Could you check a few things on this model? Use its own coordinates, in mm. Face numbers are marked on the shaded views. Round coordinates to 2 decimals unless told otherwise and drop trailing zeros. Order: outer loops, then holes, each group sorted by start corner. A loop starts at its lowest first (then second) coordinate and runs counter-clockwise, first axis right, second up. Notation, with made-up numbers: M 22,37 L 41,37 A37 cw 41,74 Z; hole C 51,74 d5. An arc over 180 degrees is marked long. Write each question's results on one line, items separated by ' | '. Start each with the question number.
1. Please list where these lines run through material, in increasing order: L1, parallel to Y at x = 0, z = 1.95; L2, parallel to Y at x = -2.25, z = 0.4; L3, parallel to Z at x = -3.75, y = 2.
2. We'd pull the mould along X, two halves only. Please class the marked faces 1, 2 and 3: released by +X, released by -X, zero draft, split by the parting line, or undercut.
3. Suppose I cut it at D-D on y = -3.75. Write out the boundary of the cut face in (x, z), and give its area (3 significant figures).
4. Suppose I cut it at C-C on z = 0.25. Write out the boundary of the cut face in (x, y).
5. Suppose I cut it at A-A on y = 0. Write out the boundary of the cut face in (x, z).
6. I'm going to push flat-ended pins straight in: pin 1 (1.5 mm diameter, centred on x = 1, z = 1.5, fed in from +Y); pin 2 (1.5 mm diameter, centred on x = 1.5, z = 1, fed in from -Y). Where does each tip first touch, or does it pass through?
Autodesk Inventor part; units mm, degrees
ref_plane "YZ Plane" through (0, 0, 0) normal (1, 0, 0) x (0, 1, 0)
ref_plane "XZ Plane" through (0, 0, 0) normal (0, 1, 0) x (-1, 0, 0)
ref_plane "XY Plane" through (0, 0, 0) normal (0, 0, 1) x (1, 0, 0)
sketch "Sketch1" plane through (0, 0, 0) normal (0, 0, 1) x (1, 0, 0)
  circle A0 centre (0, 0) radius 4
  dimension "d0" = 8
extrude "Extrusion1" add sketch "Sketch1" along normal blind 2
sketch "Sketch2" plane through (0, 0, 2) normal (0, 0, 1) x (1, 0, 0)
  circle A0 centre (0, 0) radius 2.5
  circle A1 centre (0, 0) radius 4.6
  dimension "d3" = 5
  dimension "d4" = 9.2
extrude "Extrusion2" add sketch "Sketch2" along normal blind 0.5 contours A0 | A1
sketch "Sketch3" plane through (0, 0, 0) normal (0, 0, -1) x (-1, 0, 0)
  circle A0 centre (0, 0) radius 2.5
  dimension "d7" = 5
extrude "Extrusion3" cut sketch "Sketch3" against normal blind 9
properties part number "Rotation End Cap"
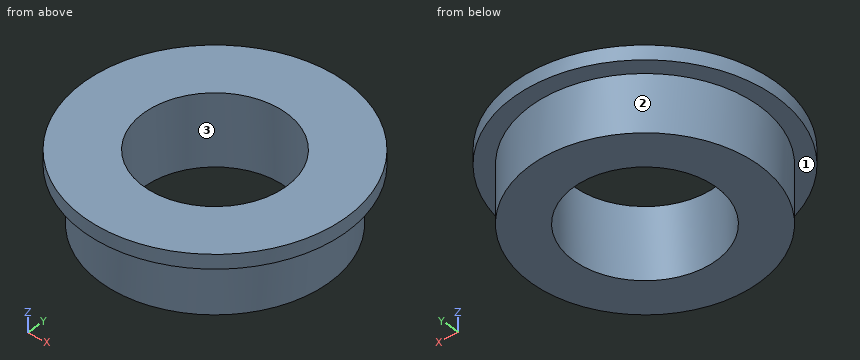
Filled sheet:
1) L1: y = -4 to -2.5, 2.5 to 4 | L2: y = -3.31 to -1.09, 1.09 to 3.31 | L3: z = 2 to 2.5
2) face 1: zero draft | face 2: split by the parting line | face 3: undercut
3) outline: M -2.66,2 L -1.39,2 L -1.39,0 L 1.39,0 L 1.39,2 L 2.66,2 L 2.66,2.5 L -2.66,2.5 Z | area: 8.23 mm^2
4) outline: C 0,0 d8; hole C 0,0 d5
5) outline: M -4.6,2 L -4,2 L -4,0 L -2.5,0 L -2.5,2.5 L -4.6,2.5 Z; M 2.5,0 L 4,0 L 4,2 L 4.6,2 L 4.6,2.5 L 2.5,2.5 Z
6) pin 1: stops at y = 4.58 | pin 2: stops at y = -3.93
